Part model, mm, in its own coordinate system. A direction names the side the tool comes from. Round coordinates to 2 decimals unless told otherwise and drop trailing zeros. Loops run counter-clockwise (first coordinate to the right, second up) from the corner with the lowest first, then second, coordinate; pieces in that order, holes last.
from build123d import *

# Parameters (mm, degrees)
SKIZZE1_W                       = 16
SKIZZE1_H                       = 16
AUFSATZ_LINEAR_AUSTRAGEN1_DEPTH = 14
SKIZZE2_W                       = 11
SKIZZE2_H                       = 7
SCHNITT_LINEAR_AUSTRAGEN1_DEPTH = 10
SKIZZE3_W                       = 7
SKIZZE3_H                       = 2
SCHNITT_LINEAR_AUSTRAGEN2_DEPTH = 10
SKIZZE4_W                       = 2
SKIZZE4_H                       = 1.6
SCHNITT_LINEAR_AUSTRAGEN3_DEPTH = 15
SKIZZE5_W                       = 16
SKIZZE5_H                       = 4
SCHNITT_LINEAR_AUSTRAGEN5_DEPTH = 1.5
SKIZZE6_W                       = 2
SKIZZE6_H                       = 2
SCHNITT_LINEAR_AUSTRAGEN6_DEPTH = 11.5


with BuildPart() as part:
    # Skizze1 → Aufsatz-Linear austragen1 (new body)
    with BuildSketch(Plane.XY):
        Rectangle(SKIZZE1_W, SKIZZE1_H)
    extrude(amount=AUFSATZ_LINEAR_AUSTRAGEN1_DEPTH)

    # Skizze2 → Schnitt-Linear austragen1 (cut)
    with BuildSketch(Plane.XZ.offset(8)):
        with Locations((0, 6.5)):
            Rectangle(SKIZZE2_W, SKIZZE2_H)
    extrude(amount=-SCHNITT_LINEAR_AUSTRAGEN1_DEPTH, mode=Mode.SUBTRACT)

    # Skizze3 → Schnitt-Linear austragen2 (cut)
    with BuildSketch(Plane.XZ.offset(8)):
        with Locations((0, 11)):
            Rectangle(SKIZZE3_W, SKIZZE3_H)
    extrude(amount=-SCHNITT_LINEAR_AUSTRAGEN2_DEPTH, mode=Mode.SUBTRACT)

    # Skizze4 → Schnitt-Linear austragen3 (cut)
    with BuildSketch(Plane.XZ.offset(8)):
        with Locations((5.1, 11.4)):
            Rectangle(SKIZZE4_W, SKIZZE4_H)
        with Locations((-5.1, 11.4)):
            Rectangle(SKIZZE4_W, SKIZZE4_H)
    extrude(amount=-SCHNITT_LINEAR_AUSTRAGEN3_DEPTH, mode=Mode.SUBTRACT)

    # Skizze5 → Schnitt-Linear austragen5 (cut)
    with BuildSketch(Plane(origin=(0, 0, 0), x_dir=(-1, 0, 0), z_dir=(0, 0, -1))):
        with Locations((0, 6)):
            Rectangle(SKIZZE5_W, SKIZZE5_H)
    extrude(amount=-SCHNITT_LINEAR_AUSTRAGEN5_DEPTH, mode=Mode.SUBTRACT)

    # Skizze6 → Schnitt-Linear austragen6 (cut)
    with BuildSketch(Plane(origin=(0, 0, 1.5), x_dir=(-1, 0, 0), z_dir=(0, 0, -1))):
        with Locations((-5.5, 6.5)):
            Rectangle(SKIZZE6_W, SKIZZE6_H)
        with Locations((5.5, 6.5)):
            Rectangle(SKIZZE6_W, SKIZZE6_H)
    extrude(amount=-SCHNITT_LINEAR_AUSTRAGEN6_DEPTH, mode=Mode.SUBTRACT)


solid = part.part
1) Tool access for faces 1 (the face through (4, -3, 10)), 2 (the face through (0, -8, 2)), 3 (the face through (6, 7, 13)): list every direction of +Z, -Z, +X, -X, +Y, -Y with a clear straight run to the whole face (end or side of a thin tool).
Values:
face 1: -Y
face 2: +Z, -Z, +X, -X, -Y
face 3: -Z
2) Mould opens along Y. For faces 4 (the face through (3.5, -3, 11)), 5 (the face through (0, 8, 8)), 6 (the face through (6.5, 6, 7)) say: released by +Y, released by -Y, zero draft, split by the parting line, or undercut.
Values:
face 4: zero draft
face 5: released by +Y
face 6: undercut
3) Slice it at D-D, the plane z = 11. Give the cut face in (x, y), then the cut area to 3 significant figures.
Values:
outline: (-8, -8) - (-6.1, -8) - (-6.1, 5.5) - (-6.5, 5.5) - (-6.5, 7.5) - (-4.5, 7.5) - (-4.5, 7) - (-4.1, 7) - (-4.1, -8) - (-3.5, -8) - (-3.5, 2) - (3.5, 2) - (3.5, -8) - (4.1, -8) - (4.1, 7) - (4.5, 7) - (4.5, 7.5) - (6.5, 7.5) - (6.5, 5.5) - (6.1, 5.5) - (6.1, -8) - (8, -8) - (8, 8) - (-8, 8) - close
area: 123 mm2
4) Drop flat-ended pins along their axis: pin 1 Ø2 at (x, z) = (0.5, 11.5) entering from -Y; pin 2 Ø0.6 at (x, z) = (-5, 8.5) entering from -Y. Give the stop position or say it passes through.
Values:
pin 1: stops at y = -8
pin 2: stops at y = 2
5) Wall check: line 1 along X through (y, z) = (5, 11.5); line 2 along X through (y, z) = (-7, 11); line 3 along X through (y, z) = (6.5, 3.75). Give the ranges that are in metal, low to high.
Values:
line 1: x = -8 to -6.1, -4.1 to 4.1, 6.1 to 8
line 2: x = -8 to -6.1, -4.1 to -3.5, 3.5 to 4.1, 6.1 to 8
line 3: x = -8 to -6.5, -4.5 to 4.5, 6.5 to 8
6) Slice it at B-B, the plane z = 2.75. Give the cut face in (x, y), then the cut area to 3 significant figures.
Values:
outline: (-8, -8) - (8, -8) - (8, 8) - (-8, 8) - close; hole (-6.5, 5.5) - (-4.5, 5.5) - (-4.5, 7.5) - (-6.5, 7.5) - close; hole (4.5, 5.5) - (6.5, 5.5) - (6.5, 7.5) - (4.5, 7.5) - close
area: 248 mm2
7) Slice it at C-C, the plane y = 4.25. Give the cut face in (x, z).
Values:
outline: (-8, 1.5) - (8, 1.5) - (8, 14) - (-8, 14) - close; hole (-6.1, 10.6) - (-4.1, 10.6) - (-4.1, 12.2) - (-6.1, 12.2) - close; hole (4.1, 10.6) - (6.1, 10.6) - (6.1, 12.2) - (4.1, 12.2) - close
8) Slice it at A-A, the plane x = -5. Give the cut face in (y, z).
Values:
outline: (-8, 0) - (4, 0) - (4, 1.5) - (5.5, 1.5) - (5.5, 10.6) - (-8, 10.6) - (-8, 10) - (2, 10) - (2, 3) - (-8, 3) - close; (-8, 12.2) - (5.5, 12.2) - (5.5, 13) - (7.5, 13) - (7.5, 1.5) - (8, 1.5) - (8, 14) - (-8, 14) - close
